from build123d import *

# Parameters (mm, degrees)
SKETCH_1_R      = 2.5
EXTRUDE_1_DEPTH = 5


with BuildPart() as part:
    # 草图1 → 凸台-拉伸1 (new body)
    with BuildSketch(Plane.XY.offset(5)):
        Polygon((50.930030436, -59.99999996), (50.930030436, 39.999999938), (35.930030436, 54.999999938), (-19.069969566, 54.999999938), (-19.069969566, 39.999999989), (-142.069969574, 39.999999989), (-142.069969574, 84.999999989), (-197.069969604, 84.999999989), (-212.069969578, 70.000000014), (-212.069969578, -90.000000037), (-197.069969604, -105.000000011), (-142.069969574, -105.000000011), (-142.069969574, -60.000000011), (-19.069969566, -60.000000011), (-19.069969566, -74.99999996), (35.930030436, -74.99999996), align=None)
        with Locations((-179.069969574, 79.999999989)):
            Circle(SKETCH_1_R, mode=Mode.SUBTRACT)
        with Locations(Location((-6.069969566, 49.999999938, 0), (0, 0, 180))):
            Circle(SKETCH_1_R, mode=Mode.SUBTRACT)
        with Locations(Location((-155.069969574, 79.999999989, 0), (0, 0, 180))):
            Circle(SKETCH_1_R, mode=Mode.SUBTRACT)
        with Locations(Location((-92.569969578, 30.000000012, 0), (0, 0, 180))):
            Circle(SKETCH_1_R, mode=Mode.SUBTRACT)
        with Locations(Location((-68.569969578, 30, 0), (0, 0, 180))):
            Circle(SKETCH_1_R, mode=Mode.SUBTRACT)
        with Locations((17.930030434, 49.999999938)):
            Circle(SKETCH_1_R, mode=Mode.SUBTRACT)
        with Locations(Location((17.930030434, -69.99999996, 0), (0, 0, 180))):
            Circle(SKETCH_1_R, mode=Mode.SUBTRACT)
        with Locations((-68.569969578, -50.000000023)):
            Circle(SKETCH_1_R, mode=Mode.SUBTRACT)
        with Locations((-92.569969578, -50.000000034)):
            Circle(SKETCH_1_R, mode=Mode.SUBTRACT)
        with Locations((-155.069969574, -100.000000011)):
            Circle(SKETCH_1_R, mode=Mode.SUBTRACT)
        with Locations((-6.069969566, -69.99999996)):
            Circle(SKETCH_1_R, mode=Mode.SUBTRACT)
        with Locations(Location((-179.069969574, -100.000000011, 0), (0, 0, 180))):
            Circle(SKETCH_1_R, mode=Mode.SUBTRACT)
    extrude(amount=-EXTRUDE_1_DEPTH)


solid = part.part
The model under review builds one solid part; all positions refer to its coordinate system, in mm. A direction names the side the tool comes from. Round coordinates to 2 decimals unless told otherwise and drop trailing zeros. Write each loop counter-clockwise with the first axis right and the second up, starting at its lowest first coordinate (ties: lowest second). Pieces come first, ordered by that corner, then holes. Notation, with made-up numbers: M -14.5,14 L 5.5,14 A23 ccw 5.5,29 Z; hole C 64,-23.5 d7. An arc over 180 degrees is marked long. Use a Markdown table: item, result. Add a question column.
Q1. We need section B-B, the plane x = -29. State the section outline as (y, z) points.
Q2. Insertion check: pin 1 (4.5 mm diameter, centred on x = -92.57, y = -50, fed in from -Z); pin 2 (2.5 mm diameter, centred on x = -76, z = 2, fed in from +Y); pin 3 (1.5 mm diameter, centred on x = -53.5, z = 2, fed in from -Y); pin 4 (2.5 mm diameter, centred on x = 0, z = 2.5, fed in from +Y). Each pin has a flat end and moves straight along its axis. Give the tip position at first contact, or say it passes through.
Q3. Machinability: for faces 4 (the face through (-80, 40, 3)), 5 (the face through (-19.07, -67, 3)), 6 (the face through (-212.07, -9, 3)), 7 (the face through (9, 55, 3)), which of the approach directions +Z, -Z, +X, -X, +Y, -Y give a long, thin tool a straight path to every point of the face, cutting with its end or side? Answer none if there is none.
Q4. To check wall thickness, follow line 1 (X direction, y = 80, z = 2.25); line 2 (X direction, y = 50, z = 2.6); line 3 (X direction, y = 66.5, z = 3.05). State the ranges of each line that lie inside material, in increasing order.
Q5. We need section C-C, the plane x = 25. State the section outline as (y, z) points.
Q6. The part is to be moulded in two halves that separate along Y. For faces 1 (the face through (-180.41, -102.11, 2.54)), 2 (the face through (-82, -9, 0)), 3 (the face through (-169, 85, 3)), say which applies: pulls with the +Y half, pulls with the -Y half, needs draft (parallel to the pull), parting line crosses it, or undercut.
Q7. We need section A-A, the plane z = 3.05. Count the separate pieces of the cut face and the enclosed holes in it, plus the area to 3 significant figures.
Findings below:
| question | item | result |
|---|---|---|
| 1 | outline | M -60,0 L 40,0 L 40,5 L -60,5 Z |
| 2 | pin 1 | passes through |
| 2 | pin 2 | stops at y = 40 |
| 2 | pin 3 | stops at y = -60 |
| 2 | pin 4 | stops at y = 55 |
| 3 | face 4 | +Z, -Z, +Y |
| 3 | face 5 | +Z, -Z, -Y |
| 3 | face 6 | +Z, -Z, -X, +Y, -Y |
| 3 | face 7 | +Z, -Z, +X, +Y |
| 4 | line 1 | x = -202.07 to -181.57, -176.57 to -157.57, -152.57 to -142.07 |
| 4 | line 2 | x = -212.07 to -142.07, -19.07 to -8.57, -3.57 to 15.43, 20.43 to 40.93 |
| 4 | line 3 | x = -212.07 to -142.07 |
| 5 | outline | M -75,0 L 55,0 L 55,5 L -75,5 Z |
| 6 | face 1 | undercut |
| 6 | face 2 | needs draft |
| 6 | face 3 | pulls with the +Y half |
| 7 | separate pieces | 1 |
| 7 | enclosed holes | 12 |
| 7 | area | 34,000 mm² |
